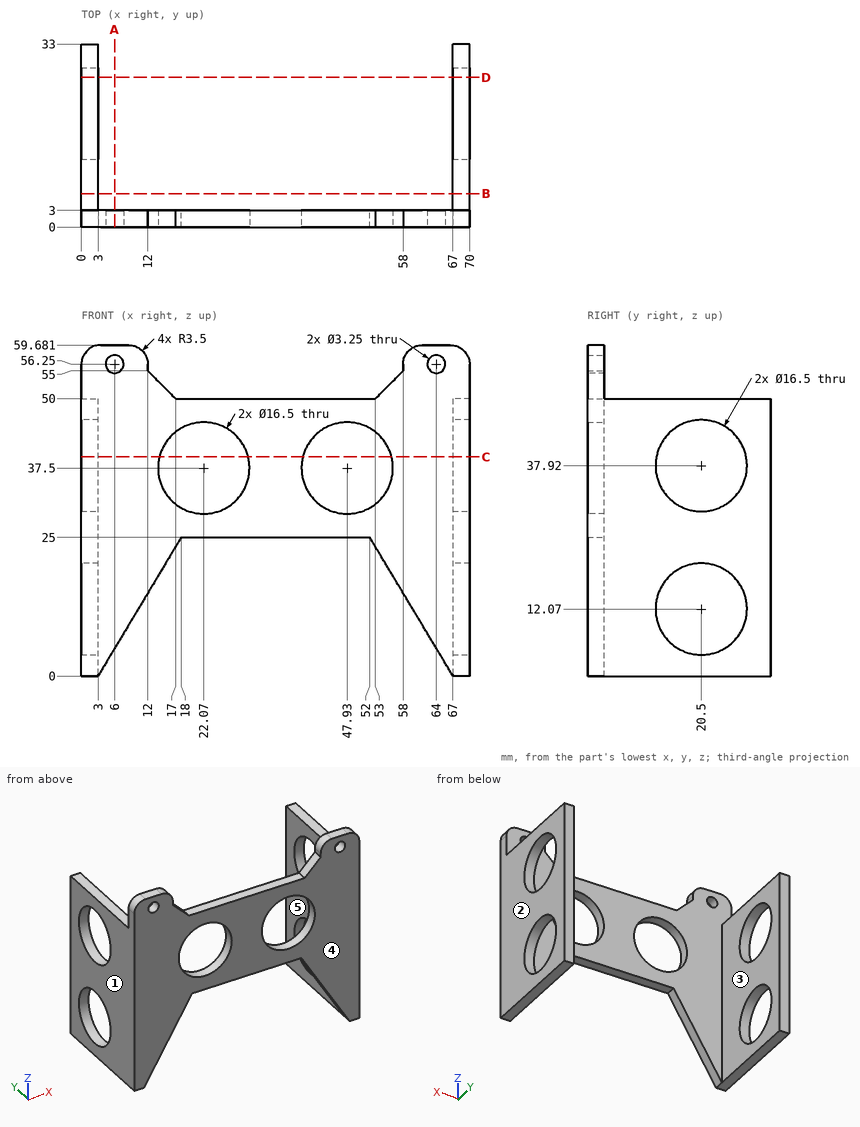
Verification items for this drawing (mm, ordinates from the low corner). A direction names the side the tool comes from. Coordinates: 2 decimals unless noted, no trailing zeros. Loops run counter-clockwise (first coordinate to the right, second up) from the corner with the lowest first, then second, coordinate; pieces in that order, holes last. Notation, with made-up numbers: (-12, 50.25) -> (2, 50.25) arc R33 ccw to (2, 82.25) -> close; hole circle Ø11 at (33, -33.5). An arc over 180 degrees is marked (long way). Put each result on its own line as item: value.
1. Section check D-D, the plane y = 27. Record the boundary of the cut face in (x, z), then the cut area to 3 significant figures.
Result set:
outline: (0, 0) -> (3, 0) -> (3, 6.99) -> (0, 6.99) -> close; (0, 17.15) -> (3, 17.15) -> (3, 32.84) -> (0, 32.84) -> close; (0, 43) -> (3, 43) -> (3, 50) -> (0, 50) -> close; (67, 0) -> (70, 0) -> (70, 6.99) -> (67, 6.99) -> close; (67, 17.15) -> (70, 17.15) -> (70, 32.84) -> (67, 32.84) -> close; (67, 43) -> (70, 43) -> (70, 50) -> (67, 50) -> close
area: 178 mm^2
2. Tool access check on the marked faces 4 and 5. Record the directions out of +Z, -Z, +X, -X, +Y, -Y that give a thin tool (end or side, any length) a straight path to the whole face; none if there is none.
Result set:
face 4: +Z, -Z, +X, -X, -Y
face 5: +Z, -Z, +Y
3. Section check B-B, the plane y = 6. Record the boundary of the cut face in (x, z), then the cut area to 3 significant figures.
Result set:
outline: (0, 0) -> (3, 0) -> (3, 50) -> (0, 50) -> close; (67, 0) -> (70, 0) -> (70, 50) -> (67, 50) -> close
area: 300 mm^2
4. Section check C-C, the plane z = 39.5. Record the boundary of the cut face in (x, y).
Result set:
outline: (0, 0) -> (14.07, 0) -> (14.07, 3) -> (3, 3) -> (3, 12.4) -> (0, 12.4) -> close; (0, 28.6) -> (3, 28.6) -> (3, 33) -> (0, 33) -> close; (30.07, 0) -> (39.93, 0) -> (39.93, 3) -> (30.07, 3) -> close; (55.93, 0) -> (70, 0) -> (70, 12.4) -> (67, 12.4) -> (67, 3) -> (55.93, 3) -> close; (67, 28.6) -> (70, 28.6) -> (70, 33) -> (67, 33) -> close
5. Mould release check, pull along X, two halves, no side actions. Record for the marked faces 1, 2 and 3: pulls with the +X half, pulls with the -X half, needs draft (parallel to the pull), parting line crosses it, or undercut.
Result set:
face 1: pulls with the -X half
face 2: pulls with the +X half
face 3: undercut
6. Section check A-A, the plane x = 6. Record the boundary of the cut face in (y, z) (1 decimal), then the cut area to 3 significant figures.
Result set:
outline: (0, 5) -> (3, 5) -> (3, 54.6) -> (0, 54.6) -> close; (0, 57.9) -> (3, 57.9) -> (3, 59.7) -> (0, 59.7) -> close
area: 154 mm^2
7. Gauge pin test, flat ends, axial feed: P1, Ø2.5, axis at x = 1.5, y = 20, coming from the +Z side; P2, Ø6, axis at x = 35.5, z = 42.5, coming from the -Y side; P3, Ø10, axis at x = 44, z = 43, coming from the +Y side; P4, Ø2.5, axis at x = 36, y = 1, coming from the -Z side. Record the tip position at first contact, or that the pin passes through.
Result set:
P1: stops at z = 50
P2: stops at y = 0
P3: stops at y = 3
P4: stops at z = 25
8. Thickness scan on line 1 (X direction, y = 1.9, z = 56.25) (1 decimal); line 2 (X direction, y = 1, z = 37) (1 decimal); line 3 (X direction, y = 5.5, z = 40). Record the ranges inside material, lowest first.
Result set:
line 1: x = 0 to 4.4, 7.6 to 12, 58 to 62.4, 65.6 to 70
line 2: x = 0 to 13.8, 30.3 to 39.7, 56.2 to 70
line 3: x = 0 to 3, 67 to 70
